from build123d import *

# Parameters (mm, degrees)
BOSS_EXTRUDE1_DEPTH  = 2.9
SOLENOID_PLACEMENT_W = 38
SOLENOID_PLACEMENT_H = 64
CUT_EXTRUDE1_DEPTH   = 104.278313309
CUT_EXTRUDE4_DEPTH   = 104.278313309
CUT_EXTRUDE5_DEPTH   = 104.278313309
SKETCH6_R            = 2.4
CUT_EXTRUDE6_DEPTH   = 104.278313309
CUT_EXTRUDE3_DEPTH   = 104.278313309
SKETCH7_W            = 10
SKETCH7_H            = 62.80248699
CUT_EXTRUDE7_DEPTH   = 99.031423533


with BuildPart() as part:
    # Sketch1 → Boss-Extrude1 (new body)
    with BuildSketch(Plane(origin=(0, 0, 0), x_dir=(1, 0, 0), z_dir=(0, 1, 0))):
        with BuildLine():
            ThreePointArc((36.856602833, -63.012624351), (0, 73), (-36.856602833, -63.012624351))
            ThreePointArc((-36.856602833, -63.012624351), (-33.368752207, -63.602994345), (-30.363140064, -61.737536127))
            ThreePointArc((-30.363140064, -61.737536127), (0, -46.75), (30.363140064, -61.737536127))
            ThreePointArc((30.363140064, -61.737536127), (33.368752207, -63.602994345), (36.856602833, -63.012624351))
        make_face()
    extrude(amount=BOSS_EXTRUDE1_DEPTH)

    # solenoid placement → Cut-Extrude1 (cut, through all)
    with BuildSketch(Plane(origin=(0, 2.9, 0), x_dir=(1, 0, 0), z_dir=(0, 1, 0))):
        with Locations((0, -4)):
            Rectangle(SOLENOID_PLACEMENT_W, SOLENOID_PLACEMENT_H)
    extrude(amount=-CUT_EXTRUDE1_DEPTH, mode=Mode.SUBTRACT)

    # Sketch4 → Cut-Extrude4 (cut, through all)
    with BuildSketch(Plane(origin=(0, 2.9, 0), x_dir=(1, 0, 0), z_dir=(0, 1, 0))):
        with BuildLine():
            Line((-13, 28), (13, 28))
            Line((13, 28), (13, 43.2))
            ThreePointArc((13, 43.2), (12.414213562, 44.614213562), (11, 45.2))
            Line((11, 45.2), (-11, 45.2))
            ThreePointArc((-11, 45.2), (-12.414213562, 44.614213562), (-13, 43.2))
            Line((-13, 43.2), (-13, 28))
        make_face()
    extrude(amount=-CUT_EXTRUDE4_DEPTH, mode=Mode.SUBTRACT)

    # Sketch5 → Cut-Extrude5 (cut, through all)
    with BuildSketch(Plane(origin=(0, 2.9, 0), x_dir=(1, 0, 0), z_dir=(0, 1, 0))):
        Polygon((-20.706882066, 48), (-23.853441033, 53.45), (-30.146558967, 53.45), (-33.293117934, 48), (-30.146558967, 42.55), (-23.853441033, 42.55), align=None)
        Polygon((23.853441033, 42.55), (20.706882066, 48), (23.853441033, 53.45), (30.146558967, 53.45), (33.293117934, 48), (30.146558967, 42.55), align=None)
    extrude(amount=-CUT_EXTRUDE5_DEPTH, mode=Mode.SUBTRACT)

    # Sketch6 → Cut-Extrude6 (cut, through all)
    with BuildSketch(Plane(origin=(0, 2.9, 0), x_dir=(1, 0, 0), z_dir=(0, 1, 0))):
        with Locations(Location((40, -40, 0), (0, 0, 270))):
            Circle(SKETCH6_R)
        with Locations(Location((-40, -40, 0), (0, 0, 270))):
            Circle(SKETCH6_R)
        with Locations(Location((-50, 40, 0), (0, 0, 270))):
            Circle(SKETCH6_R)
        with Locations(Location((50, 40, 0), (0, 0, 270))):
            Circle(SKETCH6_R)
    extrude(amount=-CUT_EXTRUDE6_DEPTH, mode=Mode.SUBTRACT)

    # Sketch3 → Cut-Extrude3 (cut, through all)
    with BuildSketch(Plane(origin=(0, 2.9, 0), x_dir=(1, 0, 0), z_dir=(0, 1, 0))):
        Polygon((-19, 28), (19, 28), (19, 32.5), (73, 32.5), (73, -32.5), (-73, -32.5), (-73, 32.5), (-19, 32.5), align=None)
    extrude(amount=-CUT_EXTRUDE3_DEPTH, mode=Mode.SUBTRACT)


with BuildPart() as cut_extrude3_piece_1:
    # of the separate pieces the step leaves, piece 1, a body of its own (cut_extrude3_pieces)
    add(part.part.solids().sort_by_distance((65.366275709, 0, -32.5))[0])


with BuildPart() as cut_extrude3_piece_2:
    # of the separate pieces the step leaves, piece 2, a body of its own (cut_extrude3_pieces)
    add(part.part.solids().sort_by_distance((-36.856602833, 0, 63.012624351))[0])

    # Sketch7 → Cut-Extrude7 (cut, through all)
    with BuildSketch(Plane(origin=(0, 2.9, 0), x_dir=(1, 0, 0), z_dir=(0, 1, 0))):
        with Locations((0, -31.401243495)):
            Rectangle(SKETCH7_W, SKETCH7_H)
    extrude(amount=-CUT_EXTRUDE7_DEPTH, mode=Mode.SUBTRACT)


with BuildPart() as cut_extrude7_piece_1:
    # of the separate pieces the step leaves, piece 1, a body of its own (cut_extrude7_pieces)
    add(cut_extrude3_piece_2.part.solids().sort_by_distance((5, 0, 47.078205475))[0])


with BuildPart() as cut_extrude7_piece_2:
    # of the separate pieces the step leaves, piece 2, a body of its own (cut_extrude7_pieces)
    add(cut_extrude3_piece_2.part.solids().sort_by_distance((-36.856602833, 0, 63.012624351))[0])


solid = cut_extrude3_piece_1.part
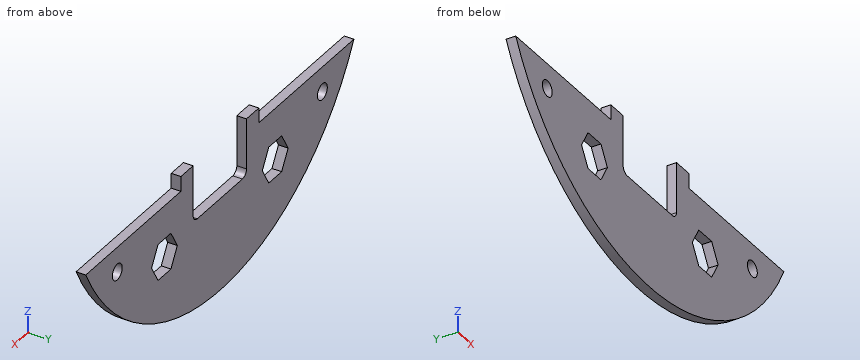
The listing builds one solid part. Answer for the finished solid, in the listing's coordinates (mm). Coordinates: 2 decimals unless noted, no trailing zeros. Loops run counter-clockwise (first coordinate to the right, second up) from the corner with the lowest first, then second, coordinate; pieces in that order, holes last. Notation, with made-up numbers: (-30.75, 37.25) -> (-13.75, 37.25) arc R30 ccw to (-13.75, 60.25) -> close; hole circle Ø2 at (74.5, 62.25). An arc over 180 degrees is marked (long way). Answer in a Markdown table with one row per item. Add a question column.
1. The part is cut by section D-D, the plane x = -22.5. Write down the section's boundary in (y, z), then the cut area to 3 significant figures.
2. The part is cut by section B-B, the plane x = 50. Write down the section's boundary in (y, z), then the cut area to 3 significant figures.
3. Consider line 1 (X direction, y = 1.8, z = -40); line 2 (X direction, y = 2.1, z = -48); line 3 (X direction, y = 2.35, z = -40.5). Determine where each line is inside the solid, lowest interval first. Write a range as [from, to].
4. Flat-ended cylindrical pins translate along their axes: P1, Ø0.9, axis at x = 26, y = 2, coming from the -Z side; P2, Ø1, axis at y = 0.5, z = -62.5, coming from the -X side; P3, Ø0.9, axis at y = 2, z = -30.5, coming from the -X side. Find the tip coordinate at first contact, or state that the pin passes through.
5. The part is cut by section A-A, the plane y = 0.8. Write down the section's boundary in (x, z).
6. The part is cut by section C-C, the plane z = -39.5. Write down the section's boundary in (x, y).
Answer below:
| question | item | result |
|---|---|---|
| 1 | outline | (0, -69.45) -> (2.9, -69.45) -> (2.9, -51.11) -> (0, -51.11) -> close; (0, -44.89) -> (2.9, -44.89) -> (2.9, -32.5) -> (0, -32.5) -> close |
| 1 | area | 89.1 mm2 |
| 2 | outline | (0, -53.19) -> (2.9, -53.19) -> (2.9, -42.4) -> (0, -42.4) -> close; (0, -37.6) -> (2.9, -37.6) -> (2.9, -32.5) -> (0, -32.5) -> close |
| 2 | area | 46.1 mm2 |
| 3 | line 1 | [-61.07, -52.4], [-47.6, -13], [13, 47.6], [52.4, 61.07] |
| 3 | line 2 | [-55, -33.29], [-20.71, 20.71], [33.29, 55] |
| 3 | line 3 | [-60.74, -52.35], [-47.65, -13], [13, 47.65], [52.35, 60.74] |
| 4 | P1 | z = -68.38 |
| 4 | P2 | x = -38.54 |
| 4 | P3 | x = -19 |
| 5 | outline | (-65.37, -32.5) arc R73 ccw to (65.37, -32.5) -> (19, -32.5) -> (19, -28) -> (13, -28) -> (13, -43.2) arc R2 cw to (11, -45.2) -> (-11, -45.2) arc R2 cw to (-13, -43.2) -> (-13, -28) -> (-19, -28) -> (-19, -32.5) -> close; hole circle Ø4.8 at (-50, -40); hole (-33.29, -48) -> (-30.15, -53.45) -> (-23.85, -53.45) -> (-20.71, -48) -> (-23.85, -42.55) -> (-30.15, -42.55) -> close; hole (20.71, -48) -> (23.85, -53.45) -> (30.15, -53.45) -> (33.29, -48) -> (30.15, -42.55) -> (23.85, -42.55) -> close; hole circle Ø4.8 at (50, -40) |
| 6 | outline | (-61.39, 0) -> (-52.35, 0) -> (-52.35, 2.9) -> (-61.39, 2.9) -> close; (-47.65, 0) -> (-13, 0) -> (-13, 2.9) -> (-47.65, 2.9) -> close; (13, 0) -> (47.65, 0) -> (47.65, 2.9) -> (13, 2.9) -> close; (52.35, 0) -> (61.39, 0) -> (61.39, 2.9) -> (52.35, 2.9) -> close |
